from build123d import *

# Parameters (mm, degrees)
SKETCH_1_R      = 6.5
SKETCH_1_R_2    = 1.5
EXTRUDE_1_DEPTH = 3
FILLET_1_R      = 5
CHAMFER_1_SIZE  = 3
FILLET_3_R      = 5
FILLET_4_R      = 2


with BuildPart() as part:
    # 草图1 → 凸台-拉伸1 (new body)
    with BuildSketch(Plane.XY):
        Polygon((15, -10), (-15, -10), (-24.5, 5), (-32.5, 5), (-32.5, 20), (-24.5, 20), (-12, 10), (12, 10), (24.5, 20), (32.5, 20), (32.5, 5), (24.5, 5), align=None)
        Circle(SKETCH_1_R, mode=Mode.SUBTRACT)
        with Locations((-29.5, 15.5)):
            Circle(SKETCH_1_R_2, mode=Mode.SUBTRACT)
        with Locations(Location((29.5, 9.5, 0), (0, 0, 180))):
            Circle(SKETCH_1_R_2, mode=Mode.SUBTRACT)
        with Locations((-29.5, 9.5)):
            Circle(SKETCH_1_R_2, mode=Mode.SUBTRACT)
        with Locations(Location((29.5, 15.5, 0), (0, 0, 180))):
            Circle(SKETCH_1_R_2, mode=Mode.SUBTRACT)
    extrude(amount=EXTRUDE_1_DEPTH)

    # 圆角1
    fillet_1_edges = [part.edges().sort_by_distance(p)[0] for p in [
        (-12, 10, 1.5),
        (12, 10, 1.5),
    ]]
    fillet(fillet_1_edges, radius=FILLET_1_R)

    # 倒角1
    chamfer_1_edges = [part.edges().sort_by_distance(p)[0] for p in [
        (15, -10, 1.5),
        (-15, -10, 1.5),
    ]]
    chamfer(chamfer_1_edges, length=CHAMFER_1_SIZE)

    # 圆角3
    fillet_3_edges = [part.edges().sort_by_distance(p)[0] for p in [
        (-24.5, 5, 1.5),
        (24.5, 5, 1.5),
    ]]
    fillet(fillet_3_edges, radius=FILLET_3_R)

    # 圆角4
    fillet_4_edges = [part.edges().sort_by_distance(p)[0] for p in [
        (-24.5, 20, 1.5),
        (24.5, 20, 1.5),
    ]]
    fillet(fillet_4_edges, radius=FILLET_4_R)


solid = part.part
The listing builds one solid part. Answer for the finished solid, in the listing's coordinates (mm). A direction names the side the tool comes from. Round coordinates to 2 decimals unless told otherwise and drop trailing zeros. Write each loop counter-clockwise with the first axis right and the second up, starting at its lowest first coordinate (ties: lowest second). Pieces come first, ordered by that corner, then holes. Notation, with made-up numbers: M 36,58.25 L 93,58.25 A18 cw 93,76.25 Z; hole C 81,-25 d3. An arc over 180 degrees is marked long. Write each question's results on one line, items separated by ' | '. Start each with the question number.
Item 1: A cutting plane is placed at D-D on z = 0.7. Write down the section's boundary in (x, y), and give its area (3 significant figures).
Item 2: A cutting plane is placed at A-A on y = -2.5. Write down the section's boundary in (x, z), and give its area (3 significant figures).
Item 3: Flat-ended cylindrical pins translate along their axes: pin 1 Ø0.9 at (x, z) = (-30.5, 1.5) entering from -Y; pin 2 Ø1.8 at (x, y) = (-29.5, 15.5) entering from +Z; pin 3 Ø1 at (x, z) = (2.5, 2) entering from +Y. Find the tip coordinate at first contact, or state that the pin passes through.
Item 4: For a pull along X with two mould halves and no side action, classify faces 1 (the face through (19.861, -2.324, 1.479)), 2 (the face through (0, -10, 1)), 3 (the face through (-31, 9.57, 1.48)) as pulls with the +X half, pulls with the -X half, needs draft (parallel to the pull), parting line crosses it, or undercut.
Item 5: Straight lines are drawn through the part: L1, parallel to Y at x = 29.5, z = 2.2; L2, parallel to Y at x = 0, z = 1.9; L3, parallel to Y at x = 10.5, z = 1.7. For each, find the intervals that lie inside material, in ascending order. Write a range as [from, to].
Item 6: For faces 4 (the face through (24.81, 4.363, 1.521)), 5 (the face through (-30, 5, 1)), 6 (the face through (-24.55, 19.89, 1.52)), determine the directions among +Z, -Z, +X, -X, +Y, -Y from which every point of the face is accessible in a straight line to the end or side of a thin tool.
Item 7: A cutting plane is placed at B-B on x = 0. Write down the section's boundary in (y, z).
Item 8: A cutting plane is placed at C-C on x = 29.5. Write down the section's boundary in (y, z).
Check sheet entries:
1) outline: M -32.5,5 L -27.25,5 A5 cw -23.03,2.68 L -16.61,-7.47 L -12,-10 L 12,-10 L 16.61,-7.47 L 23.03,2.68 A5 cw 27.25,5 L 32.5,5 L 32.5,20 L 25.2,20 A2 ccw 23.95,19.56 L 13.37,11.1 A5 cw 10.25,10 L -10.25,10 A5 cw -13.37,11.1 L -23.95,19.56 A2 ccw -25.2,20 L -32.5,20 Z; hole C -29.5,9.5 d3; hole C -29.5,15.5 d3; hole C 0,0 d13; hole C 29.5,9.5 d3; hole C 29.5,15.5 d3 | area: 1,040 mm²
2) outline: M -19.75,0 L -6,0 L -6,3 L -19.75,3 Z; M 6,0 L 19.75,0 L 19.75,3 L 6,3 Z | area: 82.5 mm²
3) pin 1: y = 5 | pin 2: through | pin 3: y = 10
4) face 1: pulls with the +X half | face 2: needs draft | face 3: undercut
5) L1: [5, 8], [11, 14], [17, 20] | L2: [-10, -6.5], [6.5, 10] | L3: [-10, 10.01]
6) face 4: +Z, -Z, +X, -Y | face 5: +Z, -Z, -X, -Y | face 6: +Z, -Z, +Y
7) outline: M -10,0 L -6.5,0 L -6.5,3 L -10,3 Z; M 6.5,0 L 10,0 L 10,3 L 6.5,3 Z
8) outline: M 5,0 L 8,0 L 8,3 L 5,3 Z; M 11,0 L 14,0 L 14,3 L 11,3 Z; M 17,0 L 20,0 L 20,3 L 17,3 Z
